from build123d import *

# Parameters (mm, degrees)
SKETCH2_R                  = 57.15
BOSS_EXTRUDE1_DEPTH        = 19.05
SKETCH3_R                  = 18.415
CUT_EXTRUDE1_DEPTH         = 16.51
SKETCH3_4_R                = 57.15
SKETCH3_4_W                = 43.18
SKETCH3_4_H                = 43.18
CUT_EXTRUDE2_DEPTH         = 12.7
SKETCH5_W                  = 114.3
SKETCH5_H                  = 114.3
CUT_EXTRUDE3_DEPTH         = 12.7
FILLET1_R                  = 27.94
F_4_0_209_DIAMETER_HOLE1_D = 5.3086


with BuildPart() as part:
    # Sketch2 → Boss-Extrude1 (new body)
    with BuildSketch(Plane(origin=(0, 0, 0), x_dir=(1, 0, 0), z_dir=(0, 1, 0))):
        with BuildLine():
            Line((-57.15, 57.15), (-57.15, -6.4e-08))
            ThreePointArc((-57.15, -6.4e-08), (-40.411152555, 40.411152534), (3.4e-08, 57.15))
            Line((3.4e-08, 57.15), (-57.15, 57.15))
        make_face()
        Circle(SKETCH2_R)
        with BuildLine():
            ThreePointArc((3.4e-08, 57.15), (40.411152557, 40.411152533), (57.15, 0))
            Line((57.15, 0), (57.15, 57.15))
            Line((57.15, 57.15), (3.4e-08, 57.15))
        make_face()
        with BuildLine():
            ThreePointArc((57.15, 0), (40.411152582, -40.411152508), (1.05e-07, -57.15))
            Line((1.05e-07, -57.15), (57.15, -57.15))
            Line((57.15, -57.15), (57.15, 0))
        make_face()
        with BuildLine():
            Line((-57.15, -6.4e-08), (-57.15, -57.15))
            Line((-57.15, -57.15), (1.05e-07, -57.15))
            ThreePointArc((1.05e-07, -57.15), (-40.411152485, -40.411152604), (-57.15, -6.4e-08))
        make_face()
    extrude(amount=BOSS_EXTRUDE1_DEPTH)

    # Sketch3 → Cut-Extrude1 (cut)
    with BuildSketch(Plane(origin=(0, 19.05, 0), x_dir=(1, 0, 0), z_dir=(0, 1, 0))):
        with Locations(Location((0, 0, 0), (0, 0, 270))):
            Circle(SKETCH3_R)
    extrude(amount=-CUT_EXTRUDE1_DEPTH, mode=Mode.SUBTRACT)

    # Sketch3<4> → Cut-Extrude2 (cut)
    with BuildSketch(Plane(origin=(0, 19.05, 0), x_dir=(1, 0, 0), z_dir=(0, 1, 0))):
        Circle(SKETCH3_4_R)
        Rectangle(SKETCH3_4_W, SKETCH3_4_H, mode=Mode.SUBTRACT)
        with BuildLine():
            Line((-57.15, -57.15), (9.5e-08, -57.15))
            ThreePointArc((9.5e-08, -57.15), (-40.411152547, -40.411152543), (-57.15, 1.01e-07))
            Line((-57.15, 1.01e-07), (-57.15, -57.15))
        make_face()
        with BuildLine():
            ThreePointArc((-57.15, 1.01e-07), (-40.411152509, 40.411152581), (0, 57.15))
            Line((0, 57.15), (-57.15, 57.15))
            Line((-57.15, 57.15), (-57.15, 1.01e-07))
        make_face()
        with BuildLine():
            ThreePointArc((0, 57.15), (40.411152545, 40.411152545), (57.15, 0))
            Line((57.15, 0), (57.15, 57.15))
            Line((57.15, 57.15), (0, 57.15))
        make_face()
        with BuildLine():
            Line((57.15, -57.15), (57.15, 0))
            ThreePointArc((57.15, 0), (40.411152578, -40.411152511), (9.5e-08, -57.15))
            Line((9.5e-08, -57.15), (57.15, -57.15))
        make_face()
    extrude(amount=-CUT_EXTRUDE2_DEPTH, mode=Mode.SUBTRACT)

    # Sketch5 → Cut-Extrude3 (cut)
    with BuildSketch(Plane(origin=(0, 6.35, 0), x_dir=(1, 0, 0), z_dir=(0, 1, 0))):
        Rectangle(SKETCH5_W, SKETCH5_H)
        with BuildLine():
            Line((21.59, 50.8), (21.59, -50.8))
            Line((21.59, -50.8), (-10.767475048, -50.8))
            ThreePointArc((-10.767475048, -50.8), (-33.401, 0), (-10.767475048, 50.8))
            Line((-10.767475048, 50.8), (21.59, 50.8))
        make_face(mode=Mode.SUBTRACT)
    extrude(amount=-CUT_EXTRUDE3_DEPTH, mode=Mode.SUBTRACT)

    # Fillet1
    fillet1_edges = [part.edges().sort_by_distance(p)[0] for p in [
        (-10.767475048, 3.175, -50.8),
        (-10.767475048, 3.175, 50.8),
    ]]
    fillet(fillet1_edges, radius=FILLET1_R)

    # #4 (0.209) Diameter Hole1 (through all)
    with Locations(Plane(origin=(0, 6.35, 0), x_dir=(1, 0, 0), z_dir=(0, 1, 0))):
        with Locations((-9.525, 34.925), (9.525, 34.925), (11.456890961, -39.511615824), (-11.456890961, -39.511615824)):
            Hole(F_4_0_209_DIAMETER_HOLE1_D / 2)


solid = part.part
CAD build for the part. Positions are in the model's coordinates, mm. A direction names the side the tool comes from. Give positions to 0.01 mm unless a question says otherwise; leave off trailing zeros. Loops run counter-clockwise (first coordinate to the right, second up) from the corner with the lowest first, then second, coordinate; pieces in that order, holes last. Notation, with made-up numbers: M -25.75,-13.5 L 9.25,-13.5 A21 ccw 9.25,-6.5 Z; hole C -39.5,72.5 d9. An arc over 180 degrees is marked long. Answer in a Markdown table with one row per item. Add a question column.
Item 1: Band-saw the part on D-D on x = 0. Give the cut face in (y, z) (3 decimals), then the cut area to 3 significant figures.
Item 2: Band-saw the part on C-C on z = -36. Give the cut face in (x, y), then the cut area to 3 significant figures.
Item 3: Probe probe 1 along X at (y, z) = (13.75, 0) (3 decimals); probe 2 along Z at (x, y) = (7.5, 4); probe 3 along Y at (x, z) = (-13, 7). List the from-to ranges inside material, lowest first.
Item 4: Mould opens along X. For faces 4 (the face through (0, 13, -21.59)), 5 (the face through (-11.22, 3.13, -47.67)), 6 (the face through (-9.5, 3.13, 37.72)) say: +X half, -X half, draft (parallel to the pull), parting line (faces both ways), or undercut.
Item 5: Band-saw the part on B-B on y = 16.5. Give the cut face in (x, z) (3 decimals).
Item 6: Drop flat-ended pins along their axis: P1, Ø18.5, axis at x = 6, z = -3.5, coming from the +Y side; P2, Ø5, axis at x = -7.5, y = 11.5, coming from the +Z side; P3, Ø5, axis at x = -9.525, z = -34.925, coming from the -Y side; P4, Ø10, axis at y = 5.5, z = -36, coming from the -X side. Give the stop position or say it passes through.
Item 7: Band-saw the part on A-A on z = 0. Give the cut face in (x, y) (3 decimals), then the cut area to 3 significant figures.
Item 8: Tool access for faces 1 (the face through (0, 13, 21.59)), 2 (the face through (0, 2.54, 0)), 3 (the face through (-21.59, 13, 0)): list every direction of +Z, -Z, +X, -X, +Y, -Y with a clear straight run to the whole face (end or side of a thin tool).
Reply:
| question | item | result |
|---|---|---|
| 1 | outline | M 0,-50.752 L 6.35,-50.752 L 6.35,-21.59 L 19.05,-21.59 L 19.05,-18.415 L 2.54,-18.415 L 2.54,18.415 L 19.05,18.415 L 19.05,21.59 L 6.35,21.59 L 6.35,50.752 L 0,50.752 Z |
| 1 | area | 585 mm^2 |
| 2 | outline | M -23.15,0 L -11.95,0 L -11.95,6.35 L -23.15,6.35 Z; M -7.1,0 L 7.1,0 L 7.1,6.35 L -7.1,6.35 Z; M 11.95,0 L 21.59,0 L 21.59,6.35 L 11.95,6.35 Z |
| 2 | area | 222 mm^2 |
| 3 | probe 1 | x = -21.59 to -18.415, 18.415 to 21.59 |
| 3 | probe 2 | z = -50.8 to -36.64, -33.21 to -16.82, 16.82 to 50.8 |
| 3 | probe 3 | y = 0 to 2.54 |
| 4 | face 4 | draft |
| 4 | face 5 | -X half |
| 4 | face 6 | undercut |
| 5 | outline | M -21.59,-21.59 L 21.59,-21.59 L 21.59,21.59 L -21.59,21.59 Z; hole C 0,0 d36.83 |
| 6 | P1 | stops at y = 2.54 |
| 6 | P2 | stops at z = 21.59 |
| 6 | P3 | passes through |
| 6 | P4 | stops at x = -25.96 |
| 7 | outline | M -33.401,0 L 21.59,0 L 21.59,19.05 L 18.415,19.05 L 18.415,2.54 L -18.415,2.54 L -18.415,19.05 L -21.59,19.05 L -21.59,6.35 L -33.401,6.35 Z |
| 7 | area | 290 mm^2 |
| 8 | face 1 | +Z, +X, -X, +Y |
| 8 | face 2 | +Y |
| 8 | face 3 | +Z, -Z, -X, +Y |
